Read the model definition and answer for the solid it produces. Units are mm, in the model's axes. A direction names the side the tool comes from. Give positions to 0.01 mm unless a question says otherwise; leave off trailing zeros. Loops run counter-clockwise (first coordinate to the right, second up) from the corner with the lowest first, then second, coordinate; pieces in that order, holes last. Notation, with made-up numbers: (-25.5, 82) - (33.5, 82) arc R19 ccw to (33.5, 98) - close; hole circle Ø3 at (-8.75, 64.5). An arc over 180 degrees is marked (long way). Write item = value, one per line.
```python
from build123d import *

# Parameters (mm, degrees)
SKETCH1_W           = 8
SKETCH1_H           = 8
SKETCH1_R           = 1.65
BOSS_EXTRUDE1_DEPTH = 3
BOSS_EXTRUDE2_DEPTH = 22
SKETCH3_R           = 13
CUT_EXTRUDE1_DEPTH  = 92.431135288
CUT_EXTRUDE3_DEPTH  = 3
SKETCH6_R           = 1.65
SKETCH6_W           = 51.3
SKETCH6_H           = 32.3
CUT_EXTRUDE4_DEPTH  = 93.198983183
BOSS_EXTRUDE4_DEPTH = 25
CUT_EXTRUDE5_DEPTH  = 93.198983183


# Read off the part's stored shape, not the designer's step: Cut-Extrude3
with BuildPart() as part:
    # Sketch1 → Boss-Extrude1 (new body)
    # profile 1 of 4: a face of its own
    with BuildSketch(Plane(origin=(0, 0, 0), x_dir=(1, 0, 0), z_dir=(0, 1, 0))):
        with BuildLine():
            Line((-18.5, 69.116947994), (-18.5, 4))
            Line((-18.5, 4), (-18.5, -4))
            Line((-18.5, -4), (-18.5, -65.642897559))
            ThreePointArc((-18.5, -65.642897559), (14.755653403, -66.584613032), (44.5, -51.681621492))
            Line((44.5, -51.681621492), (44.5, -28))
            Line((44.5, -28), (44.5, -20))
            Line((44.5, -20), (44.5, 20))
            Line((44.5, 20), (44.5, 28))
            Line((44.5, 28), (44.5, 55))
            Line((44.5, 55), (44.5, 56.028140251))
            ThreePointArc((44.5, 56.028140251), (14.554354058, 70.054073957), (-18.5, 69.116947994))
        make_face()
    # profile 2 of 4: a face of its own
    with BuildSketch(Plane(origin=(0, 0, 0), x_dir=(1, 0, 0), z_dir=(0, 1, 0))):
        with Locations((-22.5, 0)):
            Rectangle(SKETCH1_W, SKETCH1_H)
        with Locations(Location((-22.5, 0, 0), (0, 0, 270))):
            Circle(SKETCH1_R, mode=Mode.SUBTRACT)
    # profile 3 of 4: a face of its own
    with BuildSketch(Plane(origin=(0, 0, 0), x_dir=(1, 0, 0), z_dir=(0, 1, 0))):
        with Locations((48.5, -24)):
            Rectangle(SKETCH1_W, SKETCH1_H)
        with Locations(Location((48.5, -24, 0), (0, 0, 270))):
            Circle(SKETCH1_R, mode=Mode.SUBTRACT)
    # profile 4 of 4: a face of its own
    with BuildSketch(Plane(origin=(0, 0, 0), x_dir=(1, 0, 0), z_dir=(0, 1, 0))):
        with Locations((48.5, 24)):
            Rectangle(SKETCH1_W, SKETCH1_H)
        with Locations(Location((48.5, 24, 0), (0, 0, 270))):
            Circle(SKETCH1_R, mode=Mode.SUBTRACT)
    extrude(amount=BOSS_EXTRUDE1_DEPTH)

    # Sketch2 → Boss-Extrude2 (add)
    with BuildSketch(Plane(origin=(0, 3, 0), x_dir=(1, 0, 0), z_dir=(0, 1, 0))):
        with BuildLine():
            Line((44.5, -42.522376462), (44.5, 42.522376462))
            ThreePointArc((44.5, 42.522376462), (42.065161183, 44.932446124), (39.5, 47.203310265))
            Line((39.5, 47.203310265), (39.5, -47.203310265))
            ThreePointArc((39.5, -47.203310265), (42.065161183, -44.932446124), (44.5, -42.522376462))
        make_face()
    extrude(amount=BOSS_EXTRUDE2_DEPTH)

    # Sketch3 → Cut-Extrude1 (cut, through all)
    with BuildSketch(Plane(origin=(0, 3, 0), x_dir=(1, 0, 0), z_dir=(0, 1, 0))):
        with Locations((-30, -20.7)):
            Circle(SKETCH3_R)
    extrude(amount=-CUT_EXTRUDE1_DEPTH, mode=Mode.SUBTRACT)

    # Cut-Extrude3 outline → Cut-Extrude3 (cut)
    with BuildSketch(Plane(origin=(0, 0, 0), x_dir=(1, 0, 0), z_dir=(0, 1, 0))):
        with BuildLine():
            Line((44.5, -51.681621492), (44.5, -42.522376462))
            ThreePointArc((44.5, -42.522376462), (42.879948374, -44.155549226), (41.2, -45.727043421))
            Line((41.2, -45.727043421), (41.2, -54.348873033))
            ThreePointArc((41.2, -54.348873033), (42.870748276, -53.040917623), (44.5, -51.681621492))
        make_face()
        with BuildLine():
            ThreePointArc((41.2, 45.727043421), (42.879948374, 44.155549226), (44.5, 42.522376462))
            Line((44.5, 42.522376462), (44.5, 56.028140251))
            ThreePointArc((44.5, 56.028140251), (42.867784957, 57.286608495), (41.2, 58.497542683))
            Line((41.2, 58.497542683), (41.2, 45.727043421))
        make_face()
        with BuildLine():
            ThreePointArc((-18.5, -65.642897559), (-16.85525465, -66.084343007), (-15.2, -66.484584679))
            Line((-15.2, -66.484584679), (-15.2, -59.091509852))
            ThreePointArc((-15.2, -59.091509852), (-16.856674237, -58.640421812), (-18.5, -58.142897559))
            Line((-18.5, -58.142897559), (-18.5, -65.642897559))
        make_face()
    extrude(amount=CUT_EXTRUDE3_DEPTH, mode=Mode.SUBTRACT)

    # Sketch6 → Cut-Extrude4 (cut, through all)
    with BuildSketch(Plane(origin=(0, 0, 0), x_dir=(1, 0, 0), z_dir=(0, 1, 0))):
        with Locations(Location((-9.25, 44.6, 0), (0, 0, 90))):
            Circle(SKETCH6_R)
        with Locations(Location((-9.25, 4.6, 0), (0, 0, 90))):
            Circle(SKETCH6_R)
        with Locations(Location((30.75, 4.6, 0), (0, 0, 90))):
            Circle(SKETCH6_R)
        with Locations(Location((30.75, 44.6, 0), (0, 0, 90))):
            Circle(SKETCH6_R)
        with Locations(Location((-9.25, -4.6, 0), (0, 0, 90))):
            Circle(SKETCH6_R)
        with Locations(Location((30.75, -4.6, 0), (0, 0, 90))):
            Circle(SKETCH6_R)
        with Locations(Location((30.75, -44.6, 0), (0, 0, 90))):
            Circle(SKETCH6_R)
        with Locations(Location((-9.25, -44.6, 0), (0, 0, 90))):
            Circle(SKETCH6_R)
        with Locations((10.75, 23.5)):
            Rectangle(SKETCH6_W, SKETCH6_H)
        with Locations((11, -23.5)):
            Rectangle(SKETCH6_W, SKETCH6_H)
    extrude(amount=CUT_EXTRUDE4_DEPTH, mode=Mode.SUBTRACT)

    # Sketch8 → Boss-Extrude4 (add)
    with BuildSketch(Plane(origin=(0, 0, 0), x_dir=(1, 0, 0), z_dir=(0, 1, 0))):
        with BuildLine():
            Line((41, 58.637893039), (41, 54.93725967))
            ThreePointArc((41, 54.93725967), (14.207393879, 67.061557238), (-15.2, 66.843567379))
            Line((-15.2, 66.843567379), (-15.2, 69.916825586))
            ThreePointArc((-15.2, 69.916825586), (14.078834464, 70.151186164), (41, 58.637893039))
        make_face()
    extrude(amount=BOSS_EXTRUDE4_DEPTH)

    # Sketch9 → Cut-Extrude5 (cut, through all)
    with BuildSketch(Plane(origin=(0, 0, 0), x_dir=(1, 0, 0), z_dir=(0, 1, 0))):
        with BuildLine():
            Line((-18.5, 58.703939391), (-18.5, 74.933190401))
            Line((-18.5, 74.933190401), (-15.2, 74.933190401))
            Line((-15.2, 74.933190401), (-15.2, 59.643629165))
            ThreePointArc((-15.2, 59.643629165), (-16.856549297, 59.196784083), (-18.5, 58.703939391))
        make_face()
    extrude(amount=CUT_EXTRUDE5_DEPTH, mode=Mode.SUBTRACT)


solid = part.part
```
1) A cutting plane is placed at A-A on x = -22.5. Determine the outline of the cut face in (y, z).
Output:
outline = (0, -4) - (3, -4) - (3, -1.65) - (0, -1.65) - close; (0, 1.65) - (3, 1.65) - (3, 4) - (0, 4) - close
2) A cutting plane is placed at C-C on x = 10.5. Determine the outline of the cut face in (y, z).
Output:
outline = (0, -70.78) - (25, -70.78) - (25, -67.74) - (3, -67.74) - (3, -39.65) - (0, -39.65) - close; (0, -7.35) - (3, -7.35) - (3, 7.35) - (0, 7.35) - close; (0, 39.65) - (3, 39.65) - (3, 67.39) - (0, 67.39) - close
3) A cutting plane is placed at B-B on z = 0. Determine the outline of the cut face in (x, y).
Output:
outline = (-26.5, 0) - (-24.15, 0) - (-24.15, 3) - (-26.5, 3) - close; (-20.85, 0) - (44.5, 0) - (44.5, 25) - (39.5, 25) - (39.5, 3) - (-20.85, 3) - close
4) Find the intervals of material crossed by probe 1 along X at (y, z) = (1.3, 4.6); probe 2 along X at (y, z) = (2, 23); probe 3 along Z at (x, y) = (21, 1.75), in increasing order.
Output:
probe_1 = -18.5 to -10.9, -7.6 to 29.1, 32.4 to 44.5
probe_2 = -17.21 to -14.65, 36.65 to 47.19, 49.81 to 52.5
probe_3 = -68.4 to -39.65, -7.35 to 7.35, 39.65 to 64.89
5) A cutting plane is placed at D-D on z = -30. Determine the outline of the cut face in (x, y), then the cut area to 3 significant figures.
Output:
outline = (-18.5, 0) - (-14.9, 0) - (-14.9, 3) - (-18.5, 3) - close; (36.4, 0) - (44.5, 0) - (44.5, 25) - (39.5, 25) - (39.5, 3) - (36.4, 3) - close
area = 145 mm²
6) A tool of negligible diameter and unlimited length cuts with its end or side. For faces 1 (the face through (-23, 1, -4)), 2 (the face through (39.5, 14, -1)), 3 (the face through (-14.9, 1, -23)), from which of +Z, -Z, +X, -X, +Y, -Y can it reach the whole face along a straight path? Write none if from no direction.
Output:
face_1 = -Z, -X, +Y, -Y
face_2 = +Z, -X, +Y
face_3 = +Y, -Y
7) Each of these flat-tipped pins is pushed along its axis until it touches: P1, Ø5, axis at y = 13, z = -52.5, coming from the -X side; P2, Ø6.5, axis at x = 50, z = -25, coming from the +Y side; P3, Ø2.5, axis at y = 2, z = 28.5, coming from the -X side. Where does it stop, or does it pass through?
Output:
P1 = 40.92
P2 = 3
P3 = -18.5
8) The mould has two halves that part along X. Classify faces 4 (the face through (42, 25, -1)), 5 (the face through (49.615, 1.479, -25.216)), 6 (the face through (41.2, 1, -52)), 7 (the face through (29.635, 1.479, -43.384)): pulls with the +X half, pulls with the -X half, needs draft (parallel to the pull), parting line crosses it, or undercut.
Output:
face_4 = needs draft
face_5 = undercut
face_6 = pulls with the +X half
face_7 = undercut
